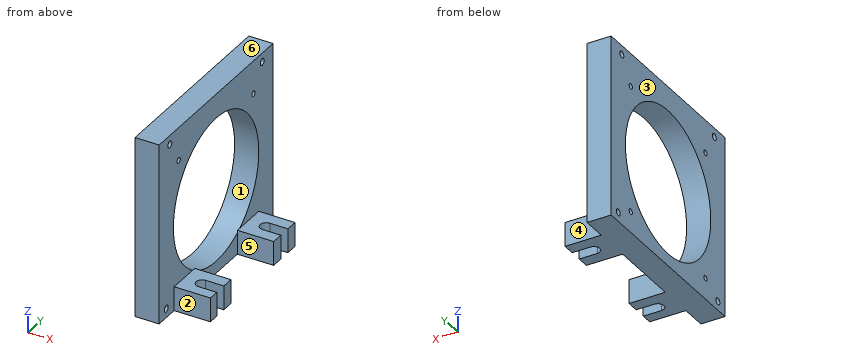
```python
from build123d import *

# Parameters (mm, degrees)
SKETCH002_W     = 160
SKETCH002_H     = 150
SKETCH002_R     = 60
PAD002_DEPTH    = 20
SKETCH005_R     = 2.25
HOLE002_DEPTH   = 25
SKETCH017_W     = 30
SKETCH017_H     = 30
SKETCH017_H_2   = 28.930618
PAD006_DEPTH    = 20
POCKET003_DEPTH = 50
SKETCH020_R     = 2.75
HOLE008_DEPTH   = 25
HOLE008_TIPS_R  = 2.75


with BuildPart() as part:
    # Sketch002 → Pad002 (new body)
    with BuildSketch(Plane.YZ.offset(500)):
        with Locations((-85, -10)):
            Rectangle(SKETCH002_W, SKETCH002_H)
        with Locations((-85, -15)):
            Circle(SKETCH002_R, mode=Mode.SUBTRACT)
    extrude(amount=PAD002_DEPTH)

    # Sketch005 → Hole002 (cut)
    with BuildSketch(Plane.YZ.offset(500)):
        with Locations((-137.5, 37.5)):
            Circle(SKETCH005_R)
        with Locations((-32.5, 37.5)):
            Circle(SKETCH005_R)
        with Locations((-32.5, -67.5)):
            Circle(SKETCH005_R)
        with Locations((-137.5, -67.5)):
            Circle(SKETCH005_R)
    extrude(amount=HOLE002_DEPTH, mode=Mode.SUBTRACT)

    # Sketch017 → Pad006 (join)
    with BuildSketch(Plane.XY.offset(-85)):
        with Locations((535, -40)):
            Rectangle(SKETCH017_W, SKETCH017_H)
        with Locations((535, -129.465309)):
            Rectangle(SKETCH017_W, SKETCH017_H_2)
    extrude(amount=PAD006_DEPTH)

    # Sketch018 → Pocket003 (cut)
    with BuildSketch(Plane.XY.offset(-85)):
        with BuildLine():
            ThreePointArc((535.000004, -35), (530.000002, -39.999999), (535.000002, -45))
            Line((535.000002, -45), (560, -45))
            ThreePointArc((560, -45), (565, -39.999999), (559.999998, -35))
            Line((535.000002, -35), (560, -35))
        make_face()
        with BuildLine():
            ThreePointArc((535.000002, -125), (530, -129.999999), (535, -135))
            Line((535, -135), (560, -135))
            ThreePointArc((560, -135), (565, -129.999999), (559.999998, -125))
            Line((535, -125), (560, -125))
        make_face()
    extrude(amount=POCKET003_DEPTH, mode=Mode.SUBTRACT)

    # Sketch020 → Hole008 (cut)
    with BuildSketch(Plane.YZ.offset(500)):
        with Locations((-155, -77.5)):
            Circle(SKETCH020_R)
        with Locations((-15, -77.5)):
            Circle(SKETCH020_R)
        with Locations((-150, 57.5)):
            Circle(SKETCH020_R)
        with Locations((-20, 57.5)):
            Circle(SKETCH020_R)
    extrude(amount=HOLE008_DEPTH, mode=Mode.SUBTRACT)

    # Hole008 tips → Hole008 tip 1 section 0
    with BuildSketch(Plane.YZ.offset(525), mode=Mode.PRIVATE) as hole008_tip_1_s0:
        with Locations((-155, -77.5)):
            Circle(HOLE008_TIPS_R)
    loft([hole008_tip_1_s0.sketch, Vertex(526.652367, -155, -77.5)], mode=Mode.SUBTRACT)

    # Hole008 tips → Hole008 tip 2 section 0
    with BuildSketch(Plane.YZ.offset(525), mode=Mode.PRIVATE) as hole008_tip_2_s0:
        with Locations((-15, -77.5)):
            Circle(HOLE008_TIPS_R)
    loft([hole008_tip_2_s0.sketch, Vertex(526.652367, -15, -77.5)], mode=Mode.SUBTRACT)

    # Hole008 tips → Hole008 tip 3 section 0
    with BuildSketch(Plane.YZ.offset(525), mode=Mode.PRIVATE) as hole008_tip_3_s0:
        with Locations((-150, 57.5)):
            Circle(HOLE008_TIPS_R)
    loft([hole008_tip_3_s0.sketch, Vertex(526.652367, -150, 57.5)], mode=Mode.SUBTRACT)

    # Hole008 tips → Hole008 tip 4 section 0
    with BuildSketch(Plane.YZ.offset(525), mode=Mode.PRIVATE) as hole008_tip_4_s0:
        with Locations((-20, 57.5)):
            Circle(HOLE008_TIPS_R)
    loft([hole008_tip_4_s0.sketch, Vertex(526.652367, -20, 57.5)], mode=Mode.SUBTRACT)


solid = part.part
```
Part model, mm, in its own coordinate system. Face numbers are marked on the shaded views. A direction names the side the tool comes from. Round coordinates to 2 decimals unless told otherwise and drop trailing zeros. Loops run counter-clockwise (first coordinate to the right, second up) from the corner with the lowest first, then second, coordinate; pieces in that order, holes last.
Item 1: Cut at C-C, the plane y = -86. Give the cut face in (x, z), then the cut area to 3 significant figures.
Item 2: Cut at A-A, the plane x = 511. State how many separate pieces and enclosed holes the cut face has, then the cut area to 3 significant figures.
Item 3: Drill centre lines: line 1 (Y direction, x = 515.5, z = -77.5); line 2 (Z direction, x = 508.75, y = -137.5); line 3 (Y direction, x = 532.5, z = -70). Where is each one in solid material? Low to high.
Item 4: Mould opens along Y. For the marked faces 1, 2 and 3 say: +Y half, -Y half, draft (parallel to the pull), parting line (faces both ways), or undercut.
Item 5: Cut at D-D, the plane y = -40. Give the cut face in (x, z).
Item 6: Drop flat-ended pins along their axis: P1, Ø22, axis at x = 534, z = -74, coming from the -Y side; P2, Ø4.5, axis at y = -20, z = 57.5, coming from the -X side; P3, Ø16.5, axis at x = 539.5, z = -71, coming from the +Y side; P4, Ø2, axis at y = -138, z = -66.5, coming from the -X side. Give the stop position or say it passes through.
Item 7: Cut at B-B, the plane z = 33. Give the cut face in (x, y).
Item 8: 3-axis set-ups, long thin cutter, end or side, ignore diameter. For the marked faces 4, 5 and 6: which of +Z, -Z, +X, -X, +Y, -Y reach the whole face in a straight line?
A:
1. outline: (500, -85) - (520, -85) - (520, -74.99) - (500, -74.99) - close; (500, 44.99) - (520, 44.99) - (520, 65) - (500, 65) - close
1. area: 600 mm2
2. separate pieces: 1
2. enclosed holes: 9
2. area: 12,500 mm2
3. line 1: y = -165 to -157.75, -152.25 to -17.75, -12.25 to -5
3. line 2: z = -85 to -69.75, -65.25 to -44.05, 14.05 to 35.25, 39.75 to 65
3. line 3: y = -143.93 to -134.33, -125.67 to -115, -55 to -44.33, -35.67 to -25
4. face 1: undercut
4. face 2: -Y half
4. face 3: draft
5. outline: (500, -85) - (530, -85) - (530, -65) - (520, -65) - (520, -54.69) - (500, -54.69) - close; (500, 24.69) - (520, 24.69) - (520, 65) - (500, 65) - close
6. P1: stops at y = -143.93
6. P2: passes through
6. P3: stops at y = -25
6. P4: stops at x = 520
7. outline: (500, -165) - (520, -165) - (520, -121) - (500, -121) - close; (500, -49) - (520, -49) - (520, -5) - (500, -5) - close
8. face 4: +Z, -Z, +X, +Y
8. face 5: +Z, -Z, +X
8. face 6: +Z, +X, -X, +Y, -Y
